Build history of the part. All positions in model axes, mm. A direction names the side the tool comes from. Round coordinates to 2 decimals unless told otherwise and drop trailing zeros. Loops run counter-clockwise (first coordinate to the right, second up) from the corner with the lowest first, then second, coordinate; pieces in that order, holes last.
from build123d import *

# Parameters (mm, degrees)
SKETCH_R        = 2.2
SKETCH_R_2      = 1.45
PAD_DEPTH       = 33
SKETCH037_R     = 2.2
SKETCH037_R_2   = 1.45
PAD016_DEPTH    = 4.5
SKETCH039_W     = 13.4
SKETCH039_H     = 10
PAD017_DEPTH    = 8
SKETCH045_W     = 20.9
SKETCH045_H     = 56.4
PAD018_DEPTH    = 34.6
POCKET022_DEPTH = 38.716621
SKETCH046_W     = 13.1
SKETCH046_H     = 26.8
POCKET023_DEPTH = 47.5
SKETCH047_R     = 1.5
POCKET024_DEPTH = 20.9
SKETCH041_W     = 3.4
SKETCH041_H     = 77.902924
POCKET025_DEPTH = 10.3
POCKET027_DEPTH = 3
FILLET014_R     = 5
FILLET015_R     = 2
FILLET016_R     = 2
FILLET017_R     = 1
POCKET028_DEPTH = 3


with BuildPart() as part:
    # Sketch → Pad (new body, symmetric)
    with BuildSketch(Plane.XZ):
        with BuildLine():
            Line((-9.25, -31.677082), (9.25, -31.677082))
            ThreePointArc((9.25, -31.677082), (23.787894, -22.872168), (32.015621, -8))
            Line((-32.015621, -8), (32.015621, -8))
            ThreePointArc((-32.015621, -8), (-23.787894, -22.872168), (-9.25, -31.677082))
        make_face()
        with Locations((24.9, -12.6)):
            Circle(SKETCH_R, mode=Mode.SUBTRACT)
        with Locations((-24.9, -12.6)):
            Circle(SKETCH_R, mode=Mode.SUBTRACT)
        with Locations((0, -12.6)):
            Circle(SKETCH_R_2, mode=Mode.SUBTRACT)
        with BuildLine():
            ThreePointArc((0, -18.243174), (-6.771568, -11.057878), (-16.248592, -13.827105))
            ThreePointArc((-16.248592, -13.827105), (-21.564175, -13.876493), (-18.494342, -18.216307))
            ThreePointArc((-18.494342, -18.216307), (-11.197344, -29.424262), (0, -22.11099))
            ThreePointArc((0, -22.11099), (18.7, -20.177082), (0, -18.243174))
        make_face(mode=Mode.SUBTRACT)
    extrude(amount=PAD_DEPTH, both=True)

    # Sketch037 → Pad016 (join)
    with BuildSketch(Plane.XZ.offset(33)):
        with BuildLine():
            ThreePointArc((-32.015621, -8), (-23.787894, -22.872168), (-9.25, -31.677082))
            Line((9.25, -31.677082), (-9.25, -31.677082))
            ThreePointArc((9.25, -31.677082), (23.787894, -22.872168), (32.015621, -8))
            Line((-32.015621, -8), (32.015621, -8))
        make_face()
        with Locations((-24.9, -12.6)):
            Circle(SKETCH037_R, mode=Mode.SUBTRACT)
        with Locations((0, -12.6)):
            Circle(SKETCH037_R_2, mode=Mode.SUBTRACT)
        with Locations((24.9, -12.6)):
            Circle(SKETCH037_R, mode=Mode.SUBTRACT)
    extrude(amount=PAD016_DEPTH)

    # Sketch039 (on Face2 of Pad016) → Pad017 (join)
    with BuildSketch(Plane(origin=(0, 0, -8), x_dir=(-1, 0, 0), z_dir=(0, 0, 1))):
        with Locations((0, 32.5)):
            Rectangle(SKETCH039_W, SKETCH039_H)
    extrude(amount=PAD017_DEPTH)

    # Sketch045 (on Face2 of Pad017) → Pad018 (join)
    with BuildSketch(Plane(origin=(0, 0, -8), x_dir=(-1, 0, 0), z_dir=(0, 0, 1))):
        with Locations((-17.15, 9.3)):
            Rectangle(SKETCH045_W, SKETCH045_H)
    extrude(amount=PAD018_DEPTH)

    # Sketch040 (on Face12 of Pad018) → Pocket022 (cut, through all)
    with BuildSketch(Plane(origin=(-6.7, 0, -11), x_dir=(0, 0, -1), z_dir=(-1, 0, 0))):
        with BuildLine():
            Line((-7.724863, 30.75), (-6.275126, 30.75))
            Line((-6.275126, 30.75), (-5.762563, 31.262563))
            ThreePointArc((-5.762563, 31.262563), (-7, 34.25), (-8.237437, 31.262563))
            Line((-7.724863, 30.75), (-8.237437, 31.262563))
        make_face()
    extrude(amount=-POCKET022_DEPTH, mode=Mode.SUBTRACT)

    # Sketch046 (on Face9 of Pocket022) → Pocket023 (cut)
    with BuildSketch(Plane(origin=(0, 18.9, 0), x_dir=(1, 0, 0), z_dir=(0, 1, 0))):
        with Locations((17.15, -9.4)):
            Rectangle(SKETCH046_W, SKETCH046_H)
    extrude(amount=-POCKET023_DEPTH, mode=Mode.SUBTRACT)

    # Sketch047 (on Face8 of Pocket023) → Pocket024 (cut)
    with BuildSketch(Plane(origin=(27.6, 0, 0), x_dir=(0, 0, 1), z_dir=(1, 0, 0))):
        with BuildLine():
            add(Edge.make_bspline(
                [(2, -18.9), (9.3, 73.1), (16.6, -18.9)],
                knots=[-7.3, -7.3, -7.3, 7.3, 7.3, 7.3], degree=2))
            Line((16.6, -18.9), (2, -18.9))
        make_face()
        with Locations((-1.5, -14.9)):
            Circle(SKETCH047_R)
        with Locations((20.1, -14.9)):
            Circle(SKETCH047_R)
    extrude(amount=-POCKET024_DEPTH, mode=Mode.SUBTRACT)

    # Sketch041 (on Face38 of Pocket024) → Pocket025 (cut)
    with BuildSketch(Plane(origin=(0, 0, 0), x_dir=(-1, 0, 0), z_dir=(0, 0, 1))):
        with Locations((0, -1.451462)):
            Rectangle(SKETCH041_W, SKETCH041_H)
    extrude(amount=-POCKET025_DEPTH, mode=Mode.SUBTRACT)

    # Sketch051 (on Face8 of Pocket025) → Pocket027 (cut)
    with BuildSketch(Plane(origin=(-6.7, 0, 0), x_dir=(0, 0, -1), z_dir=(-1, 0, 0))):
        Polygon((5.674316, 29.6), (7.348632, 32.5), (5.674316, 35.4), (2.325684, 35.4), (0.651368, 32.5), (2.325684, 29.6), align=None)
    extrude(amount=-POCKET027_DEPTH, mode=Mode.SUBTRACT)

    # Fillet014
    fillet014_edges = [part.edges().sort_by_distance(p)[0] for p in [
        (-4.2, -27.5, -8),
        (4.2, -27.5, -8),
    ]]
    fillet(fillet014_edges, radius=FILLET014_R)

    # Fillet015
    fillet015_edges = [part.edges().sort_by_distance(p)[0] for p in [
        (-4.2, -27.5, 0),
        (4.2, -27.5, 0),
    ]]
    fillet(fillet015_edges, radius=FILLET015_R)

    # Fillet016
    fillet016_edges = [part.edges().sort_by_distance(p)[0] for p in [
        (17.15, 18.9, -8),
        (17.15, 18.9, 26.6),
    ]]
    fillet(fillet016_edges, radius=FILLET016_R)

    # Fillet017
    fillet017_edges = [part.edges().sort_by_distance(p)[0] for p in [
        (25.65, 18.9, 2),
        (8.65, 18.9, 2),
        (8.65, 18.9, 16.6),
        (25.65, 18.9, 16.6),
    ]]
    fillet(fillet017_edges, radius=FILLET017_R)

    # Sketch052 (on Face18 of Fillet017) → Pocket028 (cut)
    with BuildSketch(Plane(origin=(27.6, 0, 0), x_dir=(0, 0, 1), z_dir=(1, 0, 0))):
        with BuildLine():
            ThreePointArc((-1.737258, 30.237259), (-3.999993, 35.7), (-6.262753, 30.237269))
            Line((-5.325483, 29.3), (-6.262753, 30.237269))
            Line((-2.674516, 29.3), (-5.325483, 29.3))
            Line((-1.737258, 30.237259), (-2.674516, 29.3))
        make_face()
    extrude(amount=-POCKET028_DEPTH, mode=Mode.SUBTRACT)


solid = part.part
(1) Probe line 1 (X direction, y = 6, z = -12); line 2 (Z direction, x = -2.6, y = -32.5); line 3 (Z direction, x = 24.9, y = -15.5). List the from-to ranges inside material, lowest first.
Responses:
line 1: x = -30.74 to -27.02, -22.78 to -13.99, -4.51 to -1.32, 1.32 to 4.51, 13.99 to 22.78, 27.02 to 30.74
line 2: z = -31.68 to -26.89, -13.46 to -5.75, -2.25 to 0
line 3: z = -21.66 to -14.8, -10.4 to 5.63, 12.97 to 26.6
(2) Slice it at C-C on y = 0.5. Count the separate pieces of the cut face and the enclosed holes in it, plus the area to 3 significant figures.
Responses:
separate pieces: 2
enclosed holes: 4
area: 828 mm2
(3) Pin check, flat tips, straight feed: P1, Ø1.5, axis at y = -24, z = 16, coming from the +X side; P2, Ø24.5, axis at x = -18.5, y = -11.5, coming from the +Z side; P3, Ø3, axis at x = -25.5, y = -23, coming from the -Z side; P4, Ø2.5, axis at y = 14.9, z = 20.1, coming from the +X side. Stop position of each tip, or through.
Responses:
P1: stops at x = 27.6
P2: stops at z = -8
P3: stops at z = -22.65
P4: passes through
(4) Slice it at B-B on x = -24. List the corners of the cut face in (y, z).
Responses:
outline: (-37.5, -22.65) - (33, -22.65) - (33, -14.61) - (-37.5, -14.61) - close; (-37.5, -10.59) - (33, -10.59) - (33, -8) - (-37.5, -8) - close
(5) Pull direction X, two halves, no side cores. Call faces 5 (the face through (24.6, -31.1, -2.6)), 6 (the face through (10.6, -10, 16)), 7 (the face through (-1.07, -1.76, -11.62)), 8 (the face through (-5.22, -31.03, -6.5)): +X half, -X half, draft (parallel to the pull), parting line (faces both ways), or undercut.
Responses:
face 5: +X half
face 6: undercut
face 7: undercut
face 8: draft
(6) Slice it at A-A on z = 20.1. List the corners of the cut face in (x, y).
Responses:
outline: (6.7, -37.5) - (27.6, -37.5) - (27.6, 13.4) - (23.7, 13.4) - (23.7, -28.6) - (10.6, -28.6) - (10.6, 13.4) - (6.7, 13.4) - close; (6.7, 16.4) - (10.6, 16.4) - (10.6, 18.9) - (6.7, 18.9) - close; (23.7, 16.4) - (27.6, 16.4) - (27.6, 18.9) - (23.7, 18.9) - close
(7) Slice it at D-D on x = 4.5. List the corners of the cut face in (y, z).
Responses:
outline: (-37.5, -31.68) - (33, -31.68) - (33, -28.35) - (-33, -28.35) - (-33, -12.01) - (33, -12.01) - (33, -8) - (-22.5, -8) arc R5 cw to (-27.5, -3) - (-27.5, -2) arc R2 ccw to (-29.5, 0) - (-37.5, 0) - close; hole (-31.26, -5.24) - (-30.75, -4.72) - (-30.75, -3.28) - (-31.26, -2.76) arc R1.75 ccw (long way) to start
(8) Which spindle directions (+Z, -Z, +X, -X, +Y, -Y) get a long thin tool onto all of the face, cutting with end or side? Do faces 1 (the face through (-1.7, -10, -9)), 2 (the face through (-5.22, -33.97, -1.5)), 3 (the face through (17, -28.6, 9)), 4 (the face through (-4.23, -28.07, -0.6)). Say none if no direction does.
Responses:
face 1: +Z, +Y, -Y
face 2: -X
face 3: +Y
face 4: +Z, -X, +Y
